Here's how the part is built. I have some questions about the finished solid (model axes, mm). A direction names the side the tool comes from. Round coordinates to 2 decimals unless told otherwise and drop trailing zeros. Write each loop counter-clockwise with the first axis right and the second up, starting at its lowest first coordinate (ties: lowest second). Pieces come first, ordered by that corner, then holes. Notation, with made-up numbers: (-39.5, 38) -> (-7.5, 38) arc R24 cw to (-7.5, 75) -> close; hole circle Ø9 at (57, 72). An arc over 180 degrees is marked (long way). Answer in a Markdown table with one row per item.
from build123d import *

# Parameters (mm, degrees)
SKETCH3_W           = 584.2
SKETCH3_H           = 279.4
SKETCH3_W_2         = 554.2
SKETCH3_H_2         = 249.4
BOSS_EXTRUDE3_DEPTH = 15
SKETCH4_W           = 15
SKETCH4_H           = 15
BOSS_EXTRUDE4_DEPTH = 101.6
SKETCH5_W           = 584.2
SKETCH5_H           = 279.4
SKETCH5_W_2         = 554.2
SKETCH5_H_2         = 249.4
BOSS_EXTRUDE6_DEPTH = 15


with BuildPart() as part:
    # Sketch3 → Boss-Extrude3 (new body)
    with BuildSketch(Plane(origin=(0, 0, 0), x_dir=(1, 0, 0), z_dir=(0, 1, 0))):
        Rectangle(SKETCH3_W, SKETCH3_H)
        Rectangle(SKETCH3_W_2, SKETCH3_H_2, mode=Mode.SUBTRACT)
    extrude(amount=BOSS_EXTRUDE3_DEPTH)

    # Sketch4 → Boss-Extrude4 (add)
    with BuildSketch(Plane(origin=(0, 15, 0), x_dir=(1, 0, 0), z_dir=(0, 1, 0))):
        with Locations((-284.6, 132.2)):
            Rectangle(SKETCH4_W, SKETCH4_H)
        with Locations((-284.6, -132.2)):
            Rectangle(SKETCH4_W, SKETCH4_H)
        with Locations((284.6, -132.2)):
            Rectangle(SKETCH4_W, SKETCH4_H)
        with Locations((284.6, 132.2)):
            Rectangle(SKETCH4_W, SKETCH4_H)
    extrude(amount=BOSS_EXTRUDE4_DEPTH)

    # Sketch5 → Boss-Extrude6 (add)
    with BuildSketch(Plane(origin=(0, 116.6, 0), x_dir=(1, 0, 0), z_dir=(0, 1, 0))):
        Rectangle(SKETCH5_W, SKETCH5_H)
        Rectangle(SKETCH5_W_2, SKETCH5_H_2, mode=Mode.SUBTRACT)
    extrude(amount=BOSS_EXTRUDE6_DEPTH)


solid = part.part
1) We'd pull the mould along X, two halves only. Please class faces 1 (the face through (-4, 7, 124.7)), 2 (the face through (-285, 15, -2)): +X half, -X half, draft (parallel to the pull), parting line (faces both ways), or undercut.
Response:
| item | result |
|---|---|
| face 1 | undercut |
| face 2 | draft |
2) I need wall thicknesses on line 1 (Z direction, x = -126.5, y = 124); line 2 (X direction, y = 119, z = -101). Which ranges of each line are inside material? Lowest first, please. Write a range as [from, to].
Response:
| item | result |
|---|---|
| line 1 | z = [-139.7, -124.7], [124.7, 139.7] |
| line 2 | x = [-292.1, -277.1], [277.1, 292.1] |
3) I want a section at B-B, the plane y = 98.5. List the corners of the cut face in (x, z) for me.
Response:
| item | result |
|---|---|
| outline | (-292.1, -139.7) -> (-277.1, -139.7) -> (-277.1, -124.7) -> (-292.1, -124.7) -> close; (-292.1, 124.7) -> (-277.1, 124.7) -> (-277.1, 139.7) -> (-292.1, 139.7) -> close; (277.1, -139.7) -> (292.1, -139.7) -> (292.1, -124.7) -> (277.1, -124.7) -> close; (277.1, 124.7) -> (292.1, 124.7) -> (292.1, 139.7) -> (277.1, 139.7) -> close |
4) Which directions (+Z, -Z, +X, -X, +Y, -Y) give clear straight access to the entire face, cutting with the end or side of a thin tool? Please do faces 3 (the face through (-4, 116.6, -132)), 4 (the face through (-4, 124, -124.7)), 5 (the face through (284, 65, 124.7)).
Response:
| item | result |
|---|---|
| face 3 | +Z, -Z |
| face 4 | +Y, -Y |
| face 5 | +X, -X |
5) I want a section at A-A, the plane z = -29. List the corners of the cut face in (x, y) for me, and give its area (3 significant figures).
Response:
| item | result |
|---|---|
| outline | (-292.1, 0) -> (-277.1, 0) -> (-277.1, 15) -> (-292.1, 15) -> close; (-292.1, 116.6) -> (-277.1, 116.6) -> (-277.1, 131.6) -> (-292.1, 131.6) -> close; (277.1, 0) -> (292.1, 0) -> (292.1, 15) -> (277.1, 15) -> close; (277.1, 116.6) -> (292.1, 116.6) -> (292.1, 131.6) -> (277.1, 131.6) -> close |
| area | 900 mm^2 |
6) For pin 1 (8 mm diameter, centred on x = -50, y = 21.5, fed in from +Z), with a flat end and sliding along its axis, tell me the tip position at first contact or that it passes through.
Response:
| item | result |
|---|---|
| pin 1 | passes through |
